```python
from build123d import *

# Parameters (mm, degrees)
SKETCH_W     = 160
SKETCH_H     = 90
SKETCH_R     = 1.5625
PAD_DEPTH    = 10
POCKET_DEPTH = 5
FILLET_R     = 20
FILLET001_R  = 30
FILLET002_R  = 3
FILLET003_R  = 1
FILLET004_R  = 1
FILLET005_R  = 1


with BuildPart() as part:
    # Sketch → Pad (new body)
    with BuildSketch(Plane.XY):
        with Locations((100, -45)):
            Rectangle(SKETCH_W, SKETCH_H)
        with Locations((175, -10)):
            Circle(SKETCH_R, mode=Mode.SUBTRACT)
        with Locations((175, -30)):
            Circle(SKETCH_R, mode=Mode.SUBTRACT)
        with Locations((25, -10)):
            Circle(SKETCH_R, mode=Mode.SUBTRACT)
        with Locations((25, -30)):
            Circle(SKETCH_R, mode=Mode.SUBTRACT)
        with BuildLine():
            ThreePointArc((95.0113, -14.9887), (92.0113, -11.9887), (89.0113, -14.9887))
            Line((89.0113, -14.9887), (89.0113, -30.9887))
            ThreePointArc((89.0113, -30.9887), (92.0113, -33.9887), (95.0113, -30.9887))
            Line((95.0113, -14.9887), (95.0113, -30.9887))
        make_face(mode=Mode.SUBTRACT)
        with BuildLine():
            ThreePointArc((88, -38.5), (68.5, -19), (49, -38.5))
            Line((49, -38.5), (49, -54.5))
            ThreePointArc((49, -54.5), (68.5, -74), (88, -54.5))
            Line((88, -38.5), (88, -54.5))
        make_face(mode=Mode.SUBTRACT)
        with BuildLine():
            ThreePointArc((95.0113, -62.0113), (92.0113, -59.0113), (89.0113, -62.0113))
            Line((89.0113, -62.0113), (89.0113, -78.0113))
            ThreePointArc((89.0113, -78.0113), (92.0113, -81.0113), (95.0113, -78.0113))
            Line((95.0113, -62.0113), (95.0113, -78.0113))
        make_face(mode=Mode.SUBTRACT)
        with BuildLine():
            ThreePointArc((47.9887, -62.0113), (44.9887, -59.0113), (41.9887, -62.0113))
            Line((41.9887, -62.0113), (41.9887, -78.0113))
            ThreePointArc((41.9887, -78.0113), (44.9887, -81.0113), (47.9887, -78.0113))
            Line((47.9887, -62.0113), (47.9887, -78.0113))
        make_face(mode=Mode.SUBTRACT)
        with BuildLine():
            ThreePointArc((47.9887, -14.9887), (44.9887, -11.9887), (41.9887, -14.9887))
            Line((41.9887, -14.9887), (41.9887, -30.9887))
            ThreePointArc((41.9887, -30.9887), (44.9887, -33.9887), (47.9887, -30.9887))
            Line((47.9887, -14.9887), (47.9887, -30.9887))
        make_face(mode=Mode.SUBTRACT)
    extrude(amount=PAD_DEPTH)

    # Sketch001 (on Face30 of Pad) → Pocket (cut)
    with BuildSketch(Plane.XY.offset(10)):
        with BuildLine():
            ThreePointArc((98.609297, -14.98945), (92.109297, -8.48945), (85.609297, -14.98945))
            Line((85.609297, -14.98945), (85.609297, -30.98945))
            ThreePointArc((85.609297, -30.98945), (92.109297, -37.48945), (98.609297, -30.98945))
            Line((98.609297, -14.98945), (98.609297, -30.98945))
        make_face()
        with BuildLine():
            ThreePointArc((51.586696, -14.98945), (45.086696, -8.48945), (38.586696, -14.98945))
            Line((38.586696, -14.98945), (38.586696, -30.98945))
            ThreePointArc((38.586696, -30.98945), (45.086696, -37.48945), (51.586696, -30.98945))
            Line((51.586696, -14.98945), (51.586696, -30.98945))
        make_face()
        with BuildLine():
            ThreePointArc((98.609297, -62.012051), (92.109297, -55.512051), (85.609297, -62.012051))
            Line((85.609297, -62.012051), (85.609297, -78.012051))
            ThreePointArc((85.609297, -78.012051), (92.109297, -84.512051), (98.609297, -78.012051))
            Line((98.609297, -62.012051), (98.609297, -78.012051))
        make_face()
        with BuildLine():
            ThreePointArc((51.586696, -62.012051), (45.086696, -55.512051), (38.586696, -62.012051))
            Line((38.586696, -62.012051), (38.586696, -78.012051))
            ThreePointArc((38.586696, -78.012051), (45.086696, -84.512051), (51.586696, -78.012051))
            Line((51.586696, -62.012051), (51.586696, -78.012051))
        make_face()
    extrude(amount=-POCKET_DEPTH, mode=Mode.SUBTRACT)

    # Fillet
    fillet_edges = [part.edges().sort_by_distance(p)[0] for p in [
        (20, -90, 5),
    ]]
    fillet(fillet_edges, radius=FILLET_R)

    # Fillet001
    fillet001_edges = [part.edges().sort_by_distance(p)[0] for p in [
        (180, -90, 5),
    ]]
    fillet(fillet001_edges, radius=FILLET001_R)

    # Fillet002
    fillet002_edges = [part.edges().sort_by_distance(p)[0] for p in [
        (20, 0, 5),
        (180, 0, 5),
    ]]
    fillet(fillet002_edges, radius=FILLET002_R)

    # Fillet003
    fillet003_edges = [part.edges().sort_by_distance(p)[0] for p in [
        (87.822355, -57.126141, 7.5),
    ]]
    fillet(fillet003_edges, radius=FILLET003_R)

    # Fillet004
    fillet004_edges = [part.edges().sort_by_distance(p)[0] for p in [
        (85.609297, -29.144684, 7.5),
        (51.586696, -28.794838, 7.5),
        (49.153433, -56.941385, 7.5),
    ]]
    fillet(fillet004_edges, radius=FILLET004_R)

    # Fillet005
    fillet005_edges = [part.edges().sort_by_distance(p)[0] for p in [
        (85.609297, -63.855316, 7.5),
        (51.586696, -64.205162, 7.5),
        (49.153223, -36.060285, 7.5),
        (87.822586, -35.875564, 7.5),
    ]]
    fillet(fillet005_edges, radius=FILLET005_R)


solid = part.part
```
The listing builds one solid part. Answer for the finished solid, in the listing's coordinates (mm). A direction names the side the tool comes from. Give positions to 0.01 mm unless a question says otherwise; leave off trailing zeros. Order: outer loops, then holes, each group sorted by start corner. A loop starts at its lowest first (then second) coordinate and runs counter-clockwise, first axis right, second up. Notation, with made-up numbers: (-3.5, -29) - (7.5, -29) arc R18 ccw to (7.5, -8) - close; hole circle Ø10 at (1, 77). An arc over 180 degrees is marked (long way). Answer in a Markdown table with one row per item. Add a question column.
Q1. The part is cut by section C-C (x = 175). Determine the outline of the cut face in (y, z).
Q2. The part is cut by section D-D (x = 65). Determine the outline of the cut face in (y, z), then the cut area to 3 significant figures.
Q3. For a pull along Y with two mould halves and no side action, classify faces 1 (the flat face through (38.587, -23, 8)), 2 (the flat face through (41.989, -23, 2)), 3 (the flat face through (99, -44, 10)), 4 (the flat face through (99, 0, 5)) as released by +Y, released by -Y, zero draft, split by the parting line, or undercut.
Q4. Which of the six approach directions +Z, -Z, +X, -X, +Y, -Y give full straight-line access (tool end or side, diameter ignored) to faces 5 (the flat face through (95.011, -70, 2)), 6 (the flat face through (99, -44, 0)), 7 (the cylindrical face through (45.23, -8.49, 7.54))?
Q5. Given P1, Ø5.5, axis at y = -66.5, z = 7, coming from the +X side; P2, Ø4, axis at y = -68, z = 1.5, coming from the +X side; P3, Ø4.5, axis at x = 47.5, y = -68.5, coming from the +Z side, each flat-ended and moving along its own axis, determine where each tip first touches the part or whether it passes through.
Q6. The part is cut by section B-B (y = -72.5). Determine the outline of the cut face in (x, z).
Q7. The part is cut by section A-A (z = 2). Give the number of separate pieces and of enclosed holes in the cut face, then the cut area to 3 significant figures.
Q8. Find the intervals of material crossed by line 1 along X through (y, z) = (-15.5, 4); line 2 along X through (y, z) = (-68, 9); line 3 along X through (y, z) = (-31, 4.25), in increasing order. Write a range as [from, to].
Determined:
| question | item | result |
|---|---|---|
| 1 | outline | (-76.58, 0) - (-31.56, 0) - (-31.56, 10) - (-76.58, 10) - close; (-28.44, 0) - (-11.56, 0) - (-11.56, 10) - (-28.44, 10) - close; (-8.44, 0) - (0, 0) - (0, 10) - (-8.44, 10) - close |
| 2 | outline | (-90, 0) - (-73.68, 0) - (-73.68, 10) - (-90, 10) - close; (-19.32, 0) - (0, 0) - (0, 10) - (-19.32, 10) - close |
| 2 | area | 356 mm² |
| 3 | face 1 | undercut |
| 3 | face 2 | undercut |
| 3 | face 3 | zero draft |
| 3 | face 4 | released by +Y |
| 4 | face 5 | +Z, -Z |
| 4 | face 6 | -Z, +X, -X, +Y, -Y |
| 4 | face 7 | +Z |
| 5 | P1 | stops at x = 179.76 |
| 5 | P2 | stops at x = 179.39 |
| 5 | P3 | stops at z = 5 |
| 6 | outline | (20.16, 0) - (41.99, 0) - (41.99, 5) - (38.59, 5) - (38.59, 10) - (20.16, 10) - close; (47.99, 0) - (61, 0) - (61, 10) - (51.59, 10) - (51.59, 5) - (47.99, 5) - close; (76, 0) - (89.01, 0) - (89.01, 5) - (85.61, 5) - (85.61, 10) - (76, 10) - close; (95.01, 0) - (177.27, 0) - (177.27, 10) - (98.61, 10) - (98.61, 5) - (95.01, 5) - close |
| 7 | separate pieces | 1 |
| 7 | enclosed holes | 9 |
| 7 | area | 11,800 mm² |
| 8 | line 1 | x = [20, 41.99], [47.99, 89.01], [95.01, 180] |
| 8 | line 2 | x = [20, 38.59], [51.59, 54.43], [82.57, 85.61], [98.61, 178.91] |
| 8 | line 3 | x = [20, 23.8], [26.2, 41.99], [47.99, 50.5], [86.5, 89.01], [95.01, 173.8], [176.2, 180] |
